```python
from build123d import *

# Parameters (mm, degrees)
BASE_FLANGE1_DEPTH = 88.9
CUT_EXTRUDE1_DEPTH = 3.175


# Read off the part's stored shape, not the designer's step: Base-Flange1
with BuildPart() as part:
    # Base-Flange1 outline → Base-Flange1 (new body)
    with BuildSketch(Plane.XY):
        with BuildLine():
            Line((2.54, -3.175), (25.4, -3.175))
            Line((25.4, -3.175), (25.4, 0))
            Line((25.4, 0), (2.54, 0))
            ThreePointArc((2.54, 0), (0.743948776, 0.743948776), (0, 2.54))
            Line((0, 2.54), (0, 25.4))
            Line((0, 25.4), (-3.175, 25.4))
            Line((-3.175, 25.4), (-3.175, 2.54))
            ThreePointArc((-3.175, 2.54), (-1.501115254, -1.501115254), (2.54, -3.175))
        make_face()
    extrude(amount=BASE_FLANGE1_DEPTH)

    # Sketch2 → Cut-Extrude1 (cut)
    with BuildSketch(Plane(origin=(0, 0, 0), x_dir=(0, 0, -1), z_dir=(1, 0, 0))):
        Polygon((-88.9, 25.4), (-88.9, 4.445), (-17.145, 25.4), align=None)
    extrude(amount=-CUT_EXTRUDE1_DEPTH, mode=Mode.SUBTRACT)


solid = part.part
```
The listing builds one solid part. Answer for the finished solid, in the listing's coordinates (mm). A direction names the side the tool comes from. Coordinates: 2 decimals unless noted, no trailing zeros. Write each loop counter-clockwise with the first axis right and the second up, starting at its lowest first coordinate (ties: lowest second). Pieces come first, ordered by that corner, then holes.
Q1. Section B-B, the plane y = 3.5 is taken. Write down the section's boundary in (x, z) (3 decimals), then the cut area to 3 significant figures.
Returned:
outline: (-3.175, 0) - (0, 0) - (0, 88.9) - (-3.175, 88.9) - close
area: 282 mm2
Q2. Section D-D, the plane z = 25.5 is taken. Write down the section's boundary in (x, y) (3 decimals), then the cut area to 3 significant figures.
Returned:
outline: (-3.175, 2.54) arc R5.715 ccw to (2.54, -3.175) - (25.4, -3.175) - (25.4, 0) - (2.54, 0) arc R2.54 cw to (0, 2.54) - (0, 22.96) - (-3.175, 22.96) - close
area: 158 mm2
Q3. Which of the six approach directions +Z, -Z, +X, -X, +Y, -Y give full straight-line access (tool end or side, diameter ignored) to faces 1 (the cylindrical face through (-1.5, -1.5, 43.8)), 2 (the flat face through (0, 11, 34))?
Returned:
face 1: +Z, -Z, -X, -Y
face 2: +Z, -Z, +X, +Y
Q4. Section A-A, the plane z = 9.5 is taken. Write down the section's boundary in (x, y) (3 decimals), then the cut area to 3 significant figures.
Returned:
outline: (-3.175, 2.54) arc R5.715 ccw to (2.54, -3.175) - (25.4, -3.175) - (25.4, 0) - (2.54, 0) arc R2.54 cw to (0, 2.54) - (0, 25.4) - (-3.175, 25.4) - close
area: 166 mm2
Q5. Given P1, Ø7, axis at y = 15, z = 35, coming from the +X side; P2, Ø5, axis at x = 18, z = 13.5, coming from the +Y side; P3, Ø8, axis at y = 20, z = 51.5, coming from the -X side, each flat-ended and moving along its own axis, determine where each tip first touches the part or whether it passes through.
Returned:
P1: stops at x = 0
P2: stops at y = 0
P3: passes through
Q6. Find the intervals of material crossed by line 1 along X through (y, z) = (8.75, 25) (3 decimals); line 2 along Y through (x, z) = (2, 47.5), in increasing order.
Returned:
line 1: x = -3.175 to 0
line 2: y = -3.15 to 0.06
